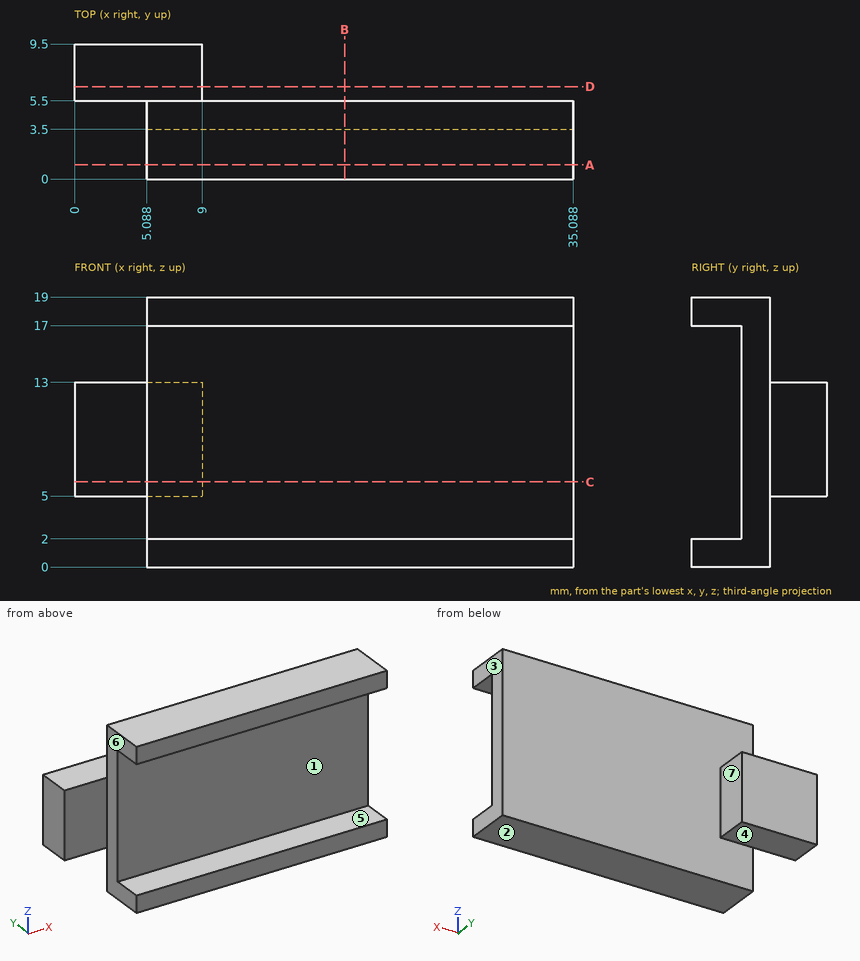
Answer from the drawing. Dimensions are ordinates in mm from the lowest x, y and z of the part. A direction names the side the tool comes from. Round coordinates to 2 decimals unless told otherwise and drop trailing zeros. Order: outer loops, then holes, each group sorted by start corner. A loop starts at its lowest first (then second) coordinate and runs counter-clockwise, first axis right, second up. Notation, with made-up numbers: (77.25, 0) - (126.25, 0) arc R12 ccw to (126.25, 9) - close; hole circle Ø2 at (45.25, 52). An arc over 180 degrees is marked (long way). Put each result on its own line as item: value. Start each with the question number.
(1) Given P1, Ø8, axis at x = 14, z = 10, coming from the -Y side; P2, Ø1.2, axis at y = 8.5, z = 9.5, coming from the +X side; P3, Ø3, axis at y = 2.5, z = 11, coming from the -X side, each flat-ended and moving along its own axis, determine where each tip first touches the part or whether it passes through.
(2) Find section C-C (z = 6). Give the vertices of the cut face in (x, y), plus the area to 3 significant figures.
(3) Straight lines are drawn through the part: probe 1 along Z at (x, y) = (13.5, 2.25); probe 2 along Y at (x, z) = (9.5, 17.75); probe 3 along Y at (x, z) = (19.5, 5). For each, find the intervals that lie inside material, in ascending order. Write a range as from..to.
(4) Find section A-A (y = 1). Give the vertices of the cut face in (x, z).
(5) For the marked faces 4, 5, 6 and 7, determine the directions among +Z, -Z, +X, -X, +Y, -Y from which every point of the face is accessible in a straight line to the end or side of a thin tool.
(6) Find section B-B (x = 19). Give the vertices of the cut face in (y, z), plus the area to 3 significant figures.
(7) Determine the mould class of the marked faces 1, 2 and 3 for opening direction Z: released by +Z, released by -Z, zero draft, split by the parting line, or undercut.
(8) Find section D-D (y = 6.5). Give the vertices of the cut face in (x, z), plus the area to 3 significant figures.
Reply:
1. P1: y = 3.5
1. P2: x = 9
1. P3: x = 5.09
2. outline: (0, 5.5) - (5.09, 5.5) - (5.09, 3.5) - (35.09, 3.5) - (35.09, 5.5) - (9, 5.5) - (9, 9.5) - (0, 9.5) - close
2. area: 96.0 mm^2
3. probe 1: 0..2, 17..19
3. probe 2: 0..5.5
3. probe 3: 3.5..5.5
4. outline: (5.09, 0) - (35.09, 0) - (35.09, 2) - (5.09, 2) - close; (5.09, 17) - (35.09, 17) - (35.09, 19) - (5.09, 19) - close
5. face 4: -Z, +X, -X, +Y
5. face 5: +X, -X, -Y
5. face 6: +Z, -Z, -X, -Y
5. face 7: +Z, -Z, +X, +Y
6. outline: (0, 0) - (5.5, 0) - (5.5, 19) - (0, 19) - (0, 17) - (3.5, 17) - (3.5, 2) - (0, 2) - close
6. area: 52.0 mm^2
7. face 1: undercut
7. face 2: released by -Z
7. face 3: zero draft
8. outline: (0, 5) - (9, 5) - (9, 13) - (0, 13) - close
8. area: 72.0 mm^2
